Could you check a few things on this model? Use its own coordinates, in mm. Round coordinates to 2 decimals unless told otherwise and drop trailing zeros. Loops run counter-clockwise (first coordinate to the right, second up) from the corner with the lowest first, then second, coordinate; pieces in that order, holes last. Notation, with made-up numbers: (8, -24) - (64, -24) arc R28 ccw to (64, 10) - close; hole circle Ø5 at (19.25, 42). An arc over 180 degrees is marked (long way). Put each result on its own line as item: value. Start each with the question number.
Autodesk Inventor part; units mm, degrees
ref_plane "YZ Plane" through (0, 0, 0) normal (1, 0, 0) x (0, 1, 0)
ref_plane "XZ Plane" through (0, 0, 0) normal (0, 1, 0) x (-1, 0, 0)
ref_plane "XY Plane" through (0, 0, 0) normal (0, 0, 1) x (1, 0, 0)
ref_plane "Work Plane1" through (0, 0, 0) normal (0, 0, 1) x (1, 0, 0)
sketch "Sketch1" plane through (0, 0, 0) normal (0, 0, 1) x (1, 0, 0)
  line L0 (-28, 30) -> (-30, 28)
  line L1 (-30, 28) -> (-30, -28)
  line L2 (-30, -28) -> (-28, -30)
  line L3 (-28, -30) -> (28, -30)
  line L4 (28, -30) -> (30, -28)
  line L5 (30, -28) -> (30, -17.7934)
  line L6 (30, 28) -> (28, 30)
  line L7 (28, 30) -> (17.7934, 30)
  line L8 (-25, -25) -> (25, -25) construction
  line L9 (25, -25) -> (25, 25) construction
  line L10 (25, 25) -> (-25, 25) construction
  line L11 (-25, 25) -> (-25, -25) construction
  line L12 (-25, -25) -> (25, 25) construction
  line L13 (25, -25) -> (-25, 25) construction
  line L14 (30, -17.7934) -> (44, -17.7934)
  line L15 (44, -9.0511) -> (44, -17.7934)
  line L16 (30, -9.0511) -> (44, -9.0511) construction
  line L17 (30, -9.0511) -> (30, 8.3051)
  line L18 (30, 8.3051) -> (44, 8.3051)
  line L19 (44, 19.2331) -> (44, 8.3051)
  line L20 (30, 19.2331) -> (44, 19.2331) construction
  line L21 (30, 28) -> (30, -28)
  line L22 (17.7934, 30) -> (17.7934, 44)
  line L23 (9.0511, 44) -> (17.7934, 44)
  line L24 (9.0511, 30) -> (9.0511, 44) construction
  line L25 (-8.3051, 30) -> (-8.3051, 44)
  line L26 (-19.2331, 44) -> (-8.3051, 44)
  line L27 (-19.2331, 30) -> (-19.2331, 44) construction
  line L28 (-19.2331, 30) -> (-28, 30)
  line L29 (30, 19.2331) -> (30, 28)
  line L30 (9.0511, 30) -> (-8.3051, 30)
  line L31 (-28, 30) -> (28, 30)
  line L32 (25, 0) -> (-25, 0)
  point P0 (0, 0)
  dimension "d0" = 50
  dimension "d1" = 50
extrude "Extrusion1" add sketch "Sketch1" along normal blind 6
sketch "Sketch2" plane through (0, 0, 6) normal (0, 0, 1) x (1, 0, 0)
  line L0 (-25, -25) -> (25, -25)
  line L1 (25, -25) -> (25, 25)
  line L2 (25, 25) -> (-25, 25)
  line L3 (-25, 25) -> (-25, -25)
  line L4 (-25, -25) -> (25, 25) construction
  line L5 (25, -25) -> (-25, 25) construction
  point P0 (0, 0)
  point P1 (25, 0)
  point P2 (-25, 0)
  point P3 (0, 25)
  point P4 (0, -25)
  dimension "d4" = 50
  dimension "d5" = 50
hole "Hole1" at (-25, 0, 6) at (25, 0, 6) direction (0, 0, -1) diameter 3.9 depth 10 tip angle 118
sketch "Sketch3" plane through (0, 0, 6) normal (0, 0, 1) x (1, 0, 0)
  circle A0 centre (25, 0) radius 1.95
  circle A1 centre (-25, 0) radius 1.95
  line L0 (-28, 30) -> (-30, 28)
  line L1 (-30, 28) -> (-30, -28)
  line L2 (-30, -28) -> (-28, -30)
  line L3 (-28, -30) -> (28, -30)
  line L4 (28, -30) -> (30, -28)
  line L5 (30, -28) -> (30, 28)
  line L6 (30, 28) -> (28, 30)
  line L7 (28, 30) -> (-28, 30)
  line L8 (-22.5, -13) -> (22.5, -13) construction
  line L9 (22.5, -13) -> (22.5, 13) construction
  line L10 (22.5, 13) -> (-22.5, 13) construction
  line L11 (-22.5, 13) -> (-22.5, -13) construction
  line L12 (-22.5, -13) -> (22.5, 13) construction
  line L13 (22.5, -13) -> (-22.5, 13) construction
  line L14 (7.5, -13) -> (-7.5, -13) construction
  line L15 (-7.5, -13) -> (-7.5, 13) construction
  line L16 (-7.5, 13) -> (7.5, 13) construction
  line L17 (7.5, 13) -> (7.5, -13) construction
  line L18 (7.5, -13) -> (-7.5, 13) construction
  line L19 (-7.5, -13) -> (7.5, 13) construction
  point P0 (0, 0)
  dimension "d13" = 45
  dimension "d14" = 26
  dimension "d15" = 15
hole "Hole2" at (22.5, 13, 6) at (7.5, 13, 6) at (-7.5, 13, 6) at (-22.5, 13, 6) at (-22.5, -13, 6) at (-7.5, -13, 6) at (7.5, -13, 6) at (22.5, -13, 6) direction (0, 0, -1) diameter 2.9 depth 10 tip angle 118 counterbore diameter 6 counterbore depth 3
properties part number "00_XY_stage-CHUO_SEIKI_LD-647-R1-Bottom"
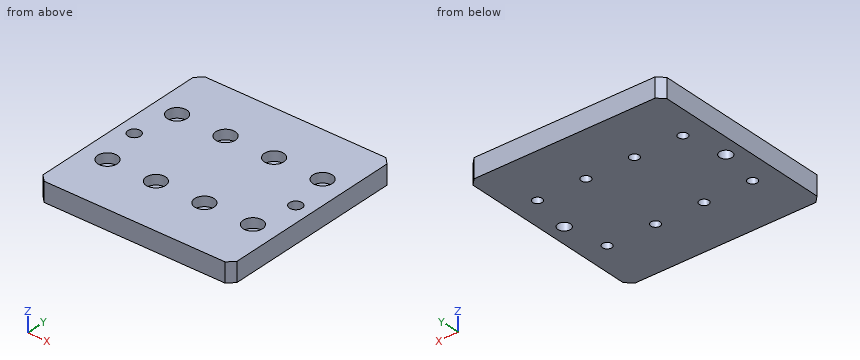
Item 1: Suppose I cut it at A-A, the plane z = 1.65. Count the separate pieces of the cut face and the enclosed holes in it, then the cut area to 3 significant figures.
Item 2: I need wall thicknesses on line 1 (Y direction, x = -7.5, z = 2.45); line 2 (X direction, y = 13, z = 1.9); line 3 (Y direction, x = -22.5, z = 4.55). Which ranges of each line are inside material? Lowest first, please. Write a range as from..to.
Item 3: Suppose I cut it at B-B, the plane x = 7.5. List the corners of the cut face in (y, z) for me.
Item 4: Will this pin go through, and if not, where does the flat tip stop? P1, Ø3, axis at x = -8.5, y = -14, coming from the +Z side.
Item 5: Suppose I cut it at C-C, the plane y = 1. List the corners of the cut face in (x, z) for me.
Numbers:
1. separate pieces: 1
1. enclosed holes: 10
1. area: 3,520 mm^2
2. line 1: -30..-14.45, -11.55..11.55, 14.45..30
2. line 2: -30..-23.95, -21.05..-8.95, -6.05..6.05, 8.95..21.05, 23.95..30
2. line 3: -30..-16, -10..10, 16..30
3. outline: (-30, 0) - (-14.45, 0) - (-14.45, 3) - (-16, 3) - (-16, 6) - (-30, 6) - close; (-11.55, 0) - (11.55, 0) - (11.55, 3) - (10, 3) - (10, 6) - (-10, 6) - (-10, 3) - (-11.55, 3) - close; (14.45, 0) - (30, 0) - (30, 6) - (16, 6) - (16, 3) - (14.45, 3) - close
4. P1: z = 3
5. outline: (-30, 0) - (-26.67, 0) - (-26.67, 6) - (-30, 6) - close; (-23.33, 0) - (23.33, 0) - (23.33, 6) - (-23.33, 6) - close; (26.67, 0) - (30, 0) - (30, 6) - (26.67, 6) - close
